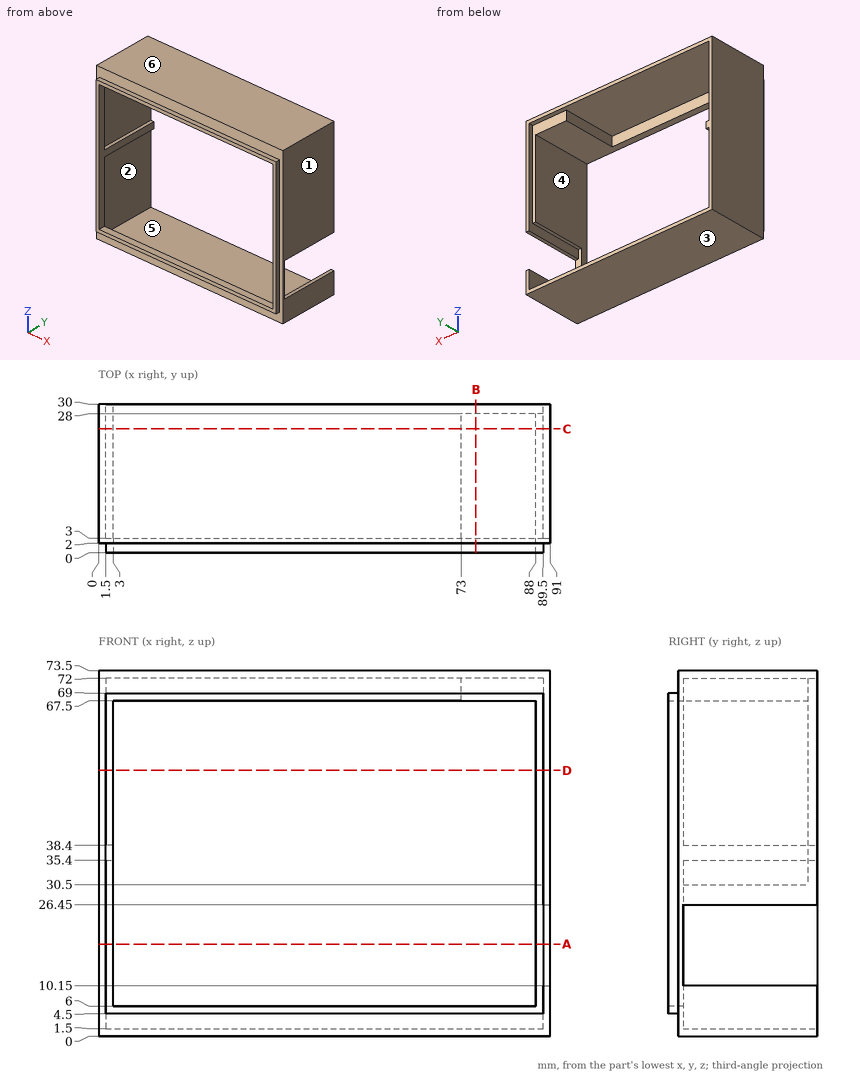
Study the drawing (mm; zero at the part's minimum x, y, z) and answer. A direction names the side the tool comes from. Round coordinates to 2 decimals unless told otherwise and drop trailing zeros. Write each loop counter-clockwise with the first axis right and the second up, starting at its lowest first coordinate (ties: lowest second). Pieces come first, ordered by that corner, then holes. Notation, with made-up numbers: (32.25, 19) - (89.25, 19) arc R8 cw to (89.25, 33) - close; hole circle Ø6 at (14, 6.5). An arc over 180 degrees is marked (long way). Use a Markdown table: item, result. Add a question column.
1. The part is cut by section A-A (z = 18.5). Write down the section's boundary in (x, y), and give its area (3 significant figures).
2. A tool of negligible diameter and unlimited length cuts with its end or side. For the marked faces 4, 5 and 6, from which of +Z, -Z, +X, -X, +Y, -Y can it reach the whole face along a straight path? Write none if from no direction.
3. Flat-ended cylindrical pins translate along their axes: P1, Ø2, axis at y = 0.5, z = 23, coming from the -X side; P2, Ø22, axis at x = 67.5, z = 46, coming from the -Y side. Find the tip coordinate at first contact, or state that the pin passes through.
4. Consider line 1 (X direction, y = 23, z = 56); line 2 (Z direction, x = 85.5, y = 15.25); line 3 (Z direction, x = 57, y = 17.75). Determine where each line is inside the solid, lowest interval first.
5. The part is cut by section D-D (z = 53.5). Write down the section's boundary in (x, y).
6. The part is cut by section C-C (y = 25). Write down the section's boundary in (x, z).
7. For a pull along X with two mould halves and no side action, classify the marked faces 1, 2 and 3 as +X half, -X half, draft (parallel to the pull), parting line (faces both ways), or undercut.
8. The part is cut by section B-B (x = 76). Write down the section's boundary in (y, z), and give its area (4 significant figures).
Reported:
| question | item | result |
|---|---|---|
| 1 | outline | (0, 2) - (1.5, 2) - (1.5, 0) - (3, 0) - (3, 3) - (1.5, 3) - (1.5, 30) - (0, 30) - close; (88, 0) - (89.5, 0) - (89.5, 2) - (91, 2) - (91, 3) - (88, 3) - close |
| 1 | area | 52.5 mm^2 |
| 2 | face 4 | +Y, -Y |
| 2 | face 5 | +Y |
| 2 | face 6 | +Z, +X, -X, +Y, -Y |
| 3 | P1 | x = 1.5 |
| 3 | P2 | through |
| 4 | line 1 | 0 to 1.5, 88 to 91 |
| 4 | line 2 | 0 to 1.5, 67.5 to 73.5 |
| 4 | line 3 | 0 to 1.5, 72 to 73.5 |
| 5 | outline | (0, 2) - (1.5, 2) - (1.5, 0) - (3, 0) - (3, 3) - (1.5, 3) - (1.5, 30) - (0, 30) - close; (88, 0) - (89.5, 0) - (89.5, 2) - (91, 2) - (91, 30) - (89.5, 30) - (89.5, 28) - (88, 28) - close |
| 6 | outline | (0, 0) - (91, 0) - (91, 10.15) - (89.5, 10.15) - (89.5, 1.5) - (1.5, 1.5) - (1.5, 35.4) - (3, 35.4) - (3, 38.4) - (1.5, 38.4) - (1.5, 72) - (73, 72) - (73, 67.5) - (88, 67.5) - (88, 30.5) - (89.5, 30.5) - (89.5, 26.45) - (91, 26.45) - (91, 73.5) - (0, 73.5) - close |
| 7 | face 1 | +X half |
| 7 | face 2 | undercut |
| 7 | face 3 | draft |
| 8 | outline | (0, 4.5) - (2, 4.5) - (2, 0) - (30, 0) - (30, 1.5) - (3, 1.5) - (3, 6) - (0, 6) - close; (0, 67.5) - (28, 67.5) - (28, 72) - (30, 72) - (30, 73.5) - (2, 73.5) - (2, 69) - (0, 69) - close |
| 8 | area | 211.5 mm^2 |
